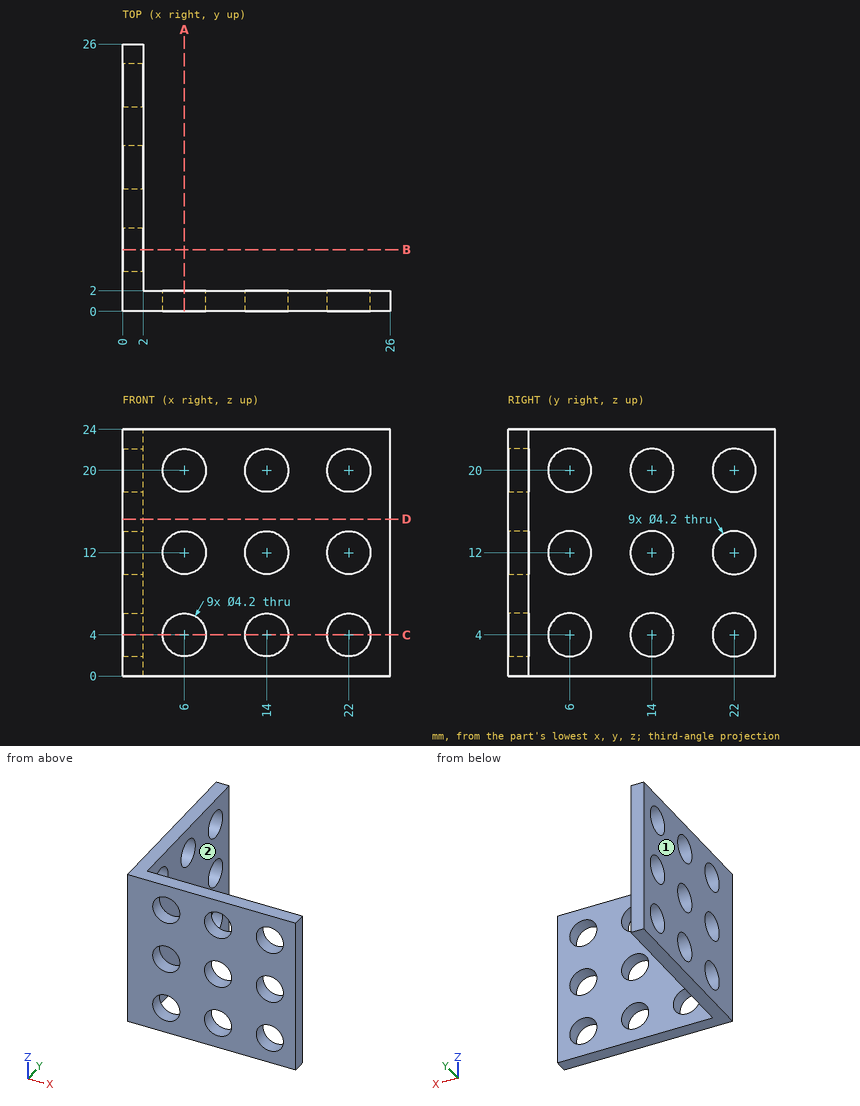
Design review of the part shown in the three views and the two pictorial views. Dimensions are in mm from the part's minimum x, y and z. A direction names the side the tool comes from. Round coordinates to 2 decimals unless told otherwise and drop trailing zeros. Loops run counter-clockwise (first coordinate to the right, second up) from the corner with the lowest first, then second, coordinate; pieces in that order, holes last.
Q1. Add section A-A on x = 6. Write out the cut boundary in (y, z), plus the area to 3 significant figures.
Result sheet:
outline: (0, 0) - (2, 0) - (2, 1.9) - (0, 1.9) - close; (0, 6.1) - (2, 6.1) - (2, 9.9) - (0, 9.9) - close; (0, 14.1) - (2, 14.1) - (2, 17.9) - (0, 17.9) - close; (0, 22.1) - (2, 22.1) - (2, 24) - (0, 24) - close
area: 22.8 mm2
Q2. Add section D-D on z = 15.25. Write out the cut boundary in (x, y).
Result sheet:
outline: (0, 0) - (26, 0) - (26, 2) - (2, 2) - (2, 26) - (0, 26) - close
Q3. To check wall thickness, follow line 1 along X through (y, z) = (0.55, 4); line 2 along Z through (x, y) = (0.7, 6); line 3 along Y through (x, z) = (16.5, 21). State the ranges of each line that lie inside material, in increasing order.
Result sheet:
line 1: x = 0 to 3.9, 8.1 to 11.9, 16.1 to 19.9, 24.1 to 26
line 2: z = 0 to 1.9, 6.1 to 9.9, 14.1 to 17.9, 22.1 to 24
line 3: y = 0 to 2
Q4. Machinability: for the marked faces 1 and 2, which of the approach directions +Z, -Z, +X, -X, +Y, -Y give a long, thin tool a straight path to every point of the face, cutting with its end or side? Answer none if there is none.
Result sheet:
face 1: +Z, -Z, -X, +Y, -Y
face 2: +Z, -Z, +X, +Y
Q5. Insertion check: pin 1 Ø5.5 at (y, z) = (6, 12) entering from +X; pin 2 Ø7 at (x, z) = (13, 9) entering from +Y. Each pin has a flat end and moves straight along its axis. Give the tip position at first contact, or say it passes through.
Result sheet:
pin 1: stops at x = 2
pin 2: stops at y = 2
Q6. Add section C-C on z = 4. Give the number of separate pieces and of enclosed holes in the cut face, plus the area to 3 significant figures.
Result sheet:
separate pieces: 7
enclosed holes: 0
area: 49.6 mm2
